CAD build for the part. Positions are in the model's coordinates, mm. A direction names the side the tool comes from. Round coordinates to 2 decimals unless told otherwise and drop trailing zeros. Write each loop counter-clockwise with the first axis right and the second up, starting at its lowest first coordinate (ties: lowest second). Pieces come first, ordered by that corner, then holes. Notation, with made-up numbers: (-30.75, 41.25) - (-4.75, 41.25) arc R20 ccw to (-4.75, 65.25) - close; hole circle Ø9 at (-4, 68.5). An arc over 180 degrees is marked (long way). Answer in a Markdown table with one row per item.
```python
from build123d import *

# Parameters (mm, degrees)
SKETCH1_W           = 50.8
SKETCH1_H           = 25.4
SKETCH1_W_2         = 47.625
SKETCH1_H_2         = 22.225
BOSS_EXTRUDE1_DEPTH = 355.6
SKETCH2_R           = 2.4892
CUT_EXTRUDE1_DEPTH  = 51.8


with BuildPart() as part:
    # Sketch1 → Boss-Extrude1 (new body)
    with BuildSketch(Plane.XY):
        with Locations((25.4, 12.7)):
            Rectangle(SKETCH1_W, SKETCH1_H)
        with Locations((25.4, 12.7)):
            Rectangle(SKETCH1_W_2, SKETCH1_H_2, mode=Mode.SUBTRACT)
    extrude(amount=BOSS_EXTRUDE1_DEPTH)

    # Sketch2 → Cut-Extrude1 (cut, through all)
    with BuildSketch(Plane(origin=(50.8, 0, 0), x_dir=(0, 0, -1), z_dir=(1, 0, 0))):
        with Locations((-342.9, 12.7)):
            Circle(SKETCH2_R)
        with Locations((-330.2, 12.7)):
            Circle(SKETCH2_R)
        with Locations((-317.5, 12.7)):
            Circle(SKETCH2_R)
        with Locations((-304.8, 12.7)):
            Circle(SKETCH2_R)
        with Locations((-292.1, 12.7)):
            Circle(SKETCH2_R)
        with Locations((-279.4, 12.7)):
            Circle(SKETCH2_R)
        with Locations((-266.7, 12.7)):
            Circle(SKETCH2_R)
        with Locations((-254, 12.7)):
            Circle(SKETCH2_R)
        with Locations((-241.3, 12.7)):
            Circle(SKETCH2_R)
        with Locations((-228.6, 12.7)):
            Circle(SKETCH2_R)
        with Locations((-215.9, 12.7)):
            Circle(SKETCH2_R)
        with Locations((-203.2, 12.7)):
            Circle(SKETCH2_R)
        with Locations((-190.5, 12.7)):
            Circle(SKETCH2_R)
        with Locations((-177.8, 12.7)):
            Circle(SKETCH2_R)
        with Locations((-165.1, 12.7)):
            Circle(SKETCH2_R)
        with Locations((-152.4, 12.7)):
            Circle(SKETCH2_R)
        with Locations((-139.7, 12.7)):
            Circle(SKETCH2_R)
        with Locations((-127, 12.7)):
            Circle(SKETCH2_R)
        with Locations((-114.3, 12.7)):
            Circle(SKETCH2_R)
        with Locations((-101.6, 12.7)):
            Circle(SKETCH2_R)
        with Locations((-88.9, 12.7)):
            Circle(SKETCH2_R)
        with Locations((-76.2, 12.7)):
            Circle(SKETCH2_R)
        with Locations((-63.5, 12.7)):
            Circle(SKETCH2_R)
        with Locations((-50.8, 12.7)):
            Circle(SKETCH2_R)
        with Locations((-38.1, 12.7)):
            Circle(SKETCH2_R)
        with Locations((-25.4, 12.7)):
            Circle(SKETCH2_R)
        with Locations((-12.7, 12.7)):
            Circle(SKETCH2_R)
    extrude(amount=-CUT_EXTRUDE1_DEPTH, mode=Mode.SUBTRACT)


solid = part.part
```
Q1. Saw through at B-B on x = 12. List the corners of the cut face in (y, z).
Computed:
| item | result |
|---|---|
| outline | (0, 0) - (1.59, 0) - (1.59, 355.6) - (0, 355.6) - close; (23.81, 0) - (25.4, 0) - (25.4, 355.6) - (23.81, 355.6) - close |
Q2. 3-axis set-ups, long thin cutter, end or side, ignore diameter. For faces 4 (the flat face through (25, 0, 175)), 5 (the flat face through (49.212, 13, 175)): which of +Z, -Z, +X, -X, +Y, -Y reach the whole face in a straight line?
Computed:
| item | result |
|---|---|
| face 4 | +Z, -Z, +X, -X, -Y |
| face 5 | +Z, -Z |
Q3. Saw through at A-A on y = 4.75. List the corners of the cut face in (x, z), then the cut area to 3 significant figures.
Computed:
| item | result |
|---|---|
| outline | (0, 0) - (1.59, 0) - (1.59, 355.6) - (0, 355.6) - close; (49.21, 0) - (50.8, 0) - (50.8, 355.6) - (49.21, 355.6) - close |
| area | 1,130 mm2 |
Q4. Drill centre lines: line 1 (Y direction, x = 38, z = 91.5); line 2 (Y direction, x = 49.95, z = 304.8); line 3 (X direction, y = 3.5, z = 156). Where is each one in solid material? Low to high.
Computed:
| item | result |
|---|---|
| line 1 | y = 0 to 1.59, 23.81 to 25.4 |
| line 2 | y = 0 to 10.21, 15.19 to 25.4 |
| line 3 | x = 0 to 1.59, 49.21 to 50.8 |
Q5. Pull direction Y, two halves, no side cores. Call faces 1 (the flat face through (25, 1.587, 175)), 2 (the flat face through (25, 25.4, 175)), 3 (the flat face through (23, 1, 0)): released by +Y, released by -Y, zero draft, split by the parting line, or undercut.
Computed:
| item | result |
|---|---|
| face 1 | undercut |
| face 2 | released by +Y |
| face 3 | zero draft |
